Here's how the part is built. I have some questions about the finished solid (model axes, mm). A direction names the side the tool comes from. Give positions to 0.01 mm unless a question says otherwise; leave off trailing zeros. Loops run counter-clockwise (first coordinate to the right, second up) from the corner with the lowest first, then second, coordinate; pieces in that order, holes last.
Q1. Suppose I cut it at D-D (x = 37.5). List the corners of the cut face in (y, z) for me, and give its area (3 significant figures).
Q2. Suppose I cut it at A-A (x = 0). List the corners of the cut face in (y, z) for me.
Q3. I'm going to push flat-ended pins straight in: P1, Ø4, axis at x = 25, y = -75, coming from the -Z side; P2, Ø4, axis at y = -32.5, z = 31, coming from the +X side; P3, Ø5, axis at x = 36, y = -64, coming from the -Z side; P4, Ø1.5, axis at y = -53.5, z = -27, coming from the +X side. Where does each tip first touch, or does it pass through?
Q4. For faces 1 (the face through (36, -76, 20.151)), 2 (the face through (0, -101.6, 40)), which set-ups out of +Z, -Z, +X, -X, +Y, -Y let a thin tool reach every point of the face, with its end or its side?
Q5. Suppose I cut it at C-C (y = -68.5). List the corners of the cut face in (x, z) for me.
Q6. Suppose I cut it at B-B (z = 0). List the corners of the cut face in (x, y) for me, and give its area (3 significant figures).
Q7. I need wall thicknesses on probe 1 along X at (y, z) = (-15, 0); probe 2 along Z at (x, y) = (-1.5, -94.5). Which ranges of each line are inside material? Lowest first, please.
```python
from build123d import *

# Parameters (mm, degrees)
F0_R     = 44.45
F0_R_2   = 38.9636
F1_DEPTH = 50.8
F3_DEPTH = 50.8


with BuildPart() as f1:
    # F0 (on Front) → F1 (new body)
    with BuildSketch(Plane.XZ):
        Circle(F0_R)
        Circle(F0_R_2, mode=Mode.SUBTRACT)
    extrude(amount=F1_DEPTH)

    # F2 (on face) → F3 (join)
    with BuildSketch(Plane.XZ.offset(50.8)):
        with BuildLine():
            Line((33.3481304372, 20.1510377228), (39.6199214877, 20.1510377228))
            ThreePointArc((39.6199214877, 20.1510377228), (0, 44.45), (-39.6199214877, 20.1510377228))
            Line((-39.6199214877, 20.1510377228), (-33.3481304372, 20.1510377228))
            ThreePointArc((-33.3481304372, 20.1510377228), (0, 38.9636), (33.3481304372, 20.1510377228))
        make_face()
    extrude(amount=F3_DEPTH)


solid = f1.part
```
Solutions:
1. outline: (-101.6, 20.15) - (-50.8, 20.15) - (-50.8, 10.58) - (0, 10.58) - (0, 23.87) - (-101.6, 23.87) - close; (-50.8, -23.87) - (0, -23.87) - (0, -10.58) - (-50.8, -10.58) - close
1. area: 1,540 mm2
2. outline: (-101.6, 38.96) - (0, 38.96) - (0, 44.45) - (-101.6, 44.45) - close; (-50.8, -44.45) - (0, -44.45) - (0, -38.96) - (-50.8, -38.96) - close
3. P1: stops at z = 28.09
3. P2: stops at x = 33.69
3. P3: stops at z = 20.15
3. P4: passes through
4. face 1: -Z, +X, -X, -Y
4. face 2: +Z, -Z, +X, -X, -Y
5. outline: (-39.62, 20.15) - (-33.35, 20.15) arc R38.96 cw to (33.35, 20.15) - (39.62, 20.15) arc R44.45 ccw to start
6. outline: (-44.45, -50.8) - (-38.96, -50.8) - (-38.96, 0) - (-44.45, 0) - close; (38.96, -50.8) - (44.45, -50.8) - (44.45, 0) - (38.96, 0) - close
6. area: 557 mm2
7. probe 1: x = -44.45 to -38.96, 38.96 to 44.45
7. probe 2: z = 38.93 to 44.42
